Build history of the part. All positions in model axes, mm. Face numbers are marked on the shaded views. A direction names the side the tool comes from. Coordinates: 2 decimals unless noted, no trailing zeros. Loops run counter-clockwise (first coordinate to the right, second up) from the corner with the lowest first, then second, coordinate; pieces in that order, holes last.
Item 1: Cut at D-D (z = 25). List the corners of the cut face in (x, y), and give its area (3 significant figures).
Item 2: Cut at C-C (z = -19). List the corners of the cut face in (x, y), and give its area (3 significant figures).
Item 3: Mould opens along X. For the marked faces 1 and 2 say: released by +X, released by -X, zero draft, split by the parting line, or undercut.
Item 4: Flat gauge pins, fed straight in: pin 1 (1 mm diameter, centred on x = 11.5, y = -3, fed in from -Z); pin 2 (4 mm diameter, centred on y = -2.5, z = 9.5, fed in from +X); pin 3 (2 mm diameter, centred on x = 13, y = -1.5, fed in from -Z). Where does each tip first touch, or does it go through?
Item 5: Cut at A-A (x = -2.5). List the corners of the cut face in (y, z).
Item 6: Drill centre lines: line 1 along Z through (x, y) = (0, -4.65) (3 decimals); line 2 along X through (y, z) = (-4.5, 14.5); line 3 along Y through (x, z) = (-3.5, 0). Where is each one in solid material? Low to high.
Item 7: Cut at B-B (z = 15). List the corners of the cut face in (x, y).
Item 8: 3-axis set-ups, long thin cutter, end or side, ignore diameter. For the marked faces 3 and 4: which of +Z, -Z, +X, -X, +Y, -Y reach the whole face in a straight line?
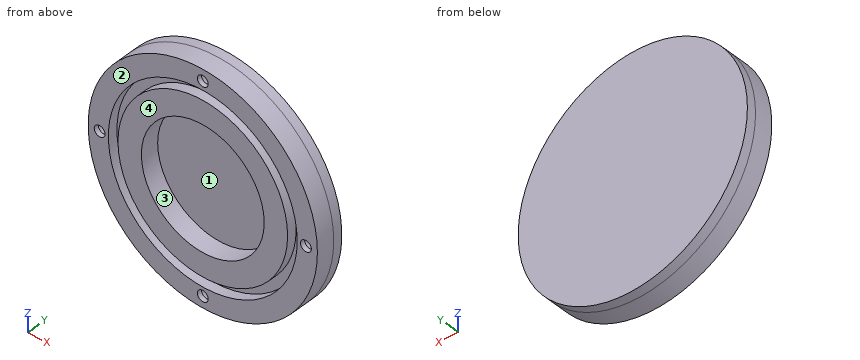
Autodesk Inventor part; units mm, degrees
ref_plane "YZ Plane" through (0, 0, 0) normal (1, 0, 0) x (0, 1, 0)
ref_plane "XZ Plane" through (0, 0, 0) normal (0, 1, 0) x (-1, 0, 0)
ref_plane "XY Plane" through (0, 0, 0) normal (0, 0, 1) x (1, 0, 0)
sketch "Sketch1" plane through (0, 0, 0) normal (0, 1, 0) x (-1, 0, 0)
  circle A0 centre (0, 0) radius 31.75
  dimension "d0" = 63.5
extrude "Extrusion1" add sketch "Sketch1" along normal blind 2.54
sketch "Sketch2" plane through (0, 0, 0) normal (0, -1, 0) x (1, 0, 0)
  circle A0 centre (0, 0) radius 31.75
  circle A1 centre (0, 0) radius 17.018
  circle A2 centre (0, 0) radius 31.75
  dimension "d4" = 34.036
extrude "Extrusion2" add sketch "Sketch2" along normal blind 5.08
sketch "Sketch3" plane through (0, -5.08, 0) normal (0, -1, 0) x (1, 0, 0)
  circle A0 centre (0, 0) radius 23.495
  circle A1 centre (0, 0) radius 17.018
  circle A2 centre (0, 0) radius 26.162
  dimension "d7" = 46.99
  dimension "d8" = 52.324
extrude "Extrusion3" cut sketch "Sketch3" against normal blind 2.667 contours A2
sketch "Sketch5" plane through (0, -5.08, 0) normal (0, -1, 0) x (1, 0, 0)
  point P0 (0, 0)
  point P1 (-28.575, 0)
  point P2 (0, -28.575)
  point P3 (28.575, 0)
  point P4 (0, 28.575)
  dimension "d18" = 28.575
  dimension "d32" = 360
hole "Hole1" at (-28.575, -5.08, 0) at (0, -5.08, 28.575) at (28.575, -5.08, 0) at (0, -5.08, -28.575) direction (0, 1, 0) diameter 3 depth 1.27 tip angle 118
properties part number "LED housing 2"
Filled sheet:
1. outline: (-19.57, -5.08) - (-7.71, -5.08) - (-7.71, -2.41) - (7.71, -2.41) - (7.71, -5.08) - (19.57, -5.08) - (19.57, 2.54) - (-19.57, 2.54) - close
1. area: 257 mm2
2. outline: (-25.44, -5.08) - (-17.98, -5.08) - (-17.98, -2.41) - (-13.82, -2.41) - (-13.82, -5.08) - (13.82, -5.08) - (13.82, -2.41) - (17.98, -2.41) - (17.98, -5.08) - (25.44, -5.08) - (25.44, 2.54) - (-25.44, 2.54) - close
2. area: 365 mm2
3. face 1: undercut
3. face 2: zero draft
4. pin 1: stops at z = -29.78
4. pin 2: stops at x = 30.85
4. pin 3: stops at z = -29.39
5. outline: (-5.08, -31.65) - (2.54, -31.65) - (2.54, 31.65) - (-5.08, 31.65) - (-5.08, 26.04) - (-2.41, 26.04) - (-2.41, 23.36) - (-5.08, 23.36) - (-5.08, 16.83) - (0, 16.83) - (0, -16.83) - (-5.08, -16.83) - (-5.08, -23.36) - (-2.41, -23.36) - (-2.41, -26.04) - (-5.08, -26.04) - close
6. line 1: z = -31.75 to -30.075, -27.075 to -26.162, -23.495 to -17.018, 17.018 to 23.495, 26.162 to 27.075, 30.075 to 31.75
6. line 2: x = -28.25 to -21.78, -18.49 to -8.91, 8.91 to 18.49, 21.78 to 28.25
6. line 3: y = 0 to 2.54
7. outline: (-27.98, -5.08) - (-21.43, -5.08) - (-21.43, -2.41) - (-18.08, -2.41) - (-18.08, -5.08) - (-8.04, -5.08) - (-8.04, 0) - (8.04, 0) - (8.04, -5.08) - (18.08, -5.08) - (18.08, -2.41) - (21.43, -2.41) - (21.43, -5.08) - (27.98, -5.08) - (27.98, 2.54) - (-27.98, 2.54) - close
8. face 3: -Y
8. face 4: +Z, -Z, +X, -X, -Y
